Could you check a few things on this model? Use its own coordinates, in mm. A direction names the side the tool comes from. Give positions to 0.01 mm unless a question says otherwise; leave off trailing zeros. Loops run counter-clockwise (first coordinate to the right, second up) from the corner with the lowest first, then second, coordinate; pieces in that order, holes last. Notation, with made-up numbers: M 82.25,-7 L 137.25,-7 A34 cw 137.25,27 Z; hole C 76.5,84 d4. An arc over 180 degrees is marked long. Return JSON: item names as keys, results as strings. Group by question number.
1. Please list where these lines run through material, in increasing order: line 1 (X direction, y = -60, z = 45); line 2 (Z direction, x = 15, y = -59); line 3 (Z direction, x = 19.5, y = -23).
2. If we mould it in two halves opening along X, with no side actions, what happens to faces 3 (the cylindrical face through (1, -37, 2)), 4 (the flat face through (15, -20, 68)), 5 (the cylindrical face through (94.06, -37.53, 1.43)), 6 (the flat face through (47, -49, 0))? For each: +X half, -X half, draft (parallel to the pull), parting line (faces both ways), or undercut.
3. For pin 1 (22 mm diameter, centred on x = 68.5, z = 61.5, fed in from -Y); pin 2 (7.5 mm diameter, centred on x = 41, z = 45.5, fed in from -Y); pin 3 (17 mm diameter, centred on x = 15, z = 45, fed in from -Y), each with a flat end and sliding along its axis, tell me the tip position at first contact or that it passes through.
4. If we section it at D-D (x = 15): Write out the boundary of the cut face in (y, z), plus the area to 3 significant figures.
5. If we section it at B-B (z = 57): Write out the boundary of the cut face in (x, y), plus the area to 3 significant figures.
6. If we section it at C-C (x = 41): Write out the boundary of the cut face in (y, z), plus the area to 3 significant figures.
7. If we section it at A-A (y = -62.5): Write out the boundary of the cut face in (x, z), plus the area to 3 significant figures.
8. For faces 1 (the flat face through (27.28, -87.13, 44.37)), 2 (the flat face through (15, -20, 45)), which set-ups out of +Z, -Z, +X, -X, +Y, -Y let a thin tool reach every point of the face, with its end or its side?
```python
from build123d import *

# Parameters (mm, degrees)
F0_W        = 95.5598546359
F0_H        = 90
F1_DEPTH    = 100
F2_R        = 5
F3_W        = 20
F3_H        = 70
F3_R        = 7.5
F4_DEPTH    = 80
F5_T1_DEPTH = 92.4997500025
F7_DEPTH    = 90
F8_T1_DEPTH = 105.435292613


# Not quite as in the source:
# - a fillet or chamfer that OpenCascade refuses, or shapes differently, is made with other operations: its cross-section is extruded or revolved along the edge and cut away or added


with BuildPart() as f1:
    # F0 (on Front) → F1 (new body)
    with BuildSketch(Plane.XZ):
        with Locations((47.7799273179, 45)):
            Rectangle(F0_W, F0_H)
    extrude(amount=F1_DEPTH)

    # F2
    f2_edges = [f1.edges().sort_by_distance(p)[0] for p in [
        (95.559855, -50, 90),
        (95.559855, -50, 0),
        (0, -50, 0),
        (0, -50, 90),
    ]]
    fillet(f2_edges, radius=F2_R)

    # F3 (on face) → F4 (cut)
    with BuildSketch(Plane.XZ.offset(100)):
        with Locations((73.0598546359, 45)):
            Rectangle(F3_W, F3_H)
        with Locations((15, 45)):
            Circle(F3_R)
        with Locations((15, 68)):
            Circle(F3_R)
        with Locations((40, 45)):
            Circle(F3_R)
        with Locations((40, 68)):
            Circle(F3_R)
        with Locations((15, 20)):
            Circle(F3_R)
        with Locations((40, 20)):
            Circle(F3_R)
    extrude(amount=-F4_DEPTH, mode=Mode.SUBTRACT)

    # F5: fillet of radius 5 on 4 edges, made by hand

    # F5_s2 → F5_t1 (join)
    with BuildSketch(Plane.XZ.offset(7.5002499975)):
        with BuildLine():
            ThreePointArc((68.0597546359, 80.0001), (64.5242207299, 78.5356339059), (63.0597546359, 75.0001))
            Line((63.0597546359, 75.0001), (62.9597546359, 75.0001))
            ThreePointArc((62.9597546359, 75.0001), (62.9598546359, 77.50005), (62.9598546359, 80))
            Line((62.9598546359, 80), (63.0598546359, 80.1))
            ThreePointArc((63.0598546359, 80.1), (65.5598046359, 80.1), (68.0597546359, 80.1001))
            Line((68.0597546359, 80.1001), (68.0597546359, 80.0001))
        make_face()
        with BuildLine():
            ThreePointArc((78.0599546359, 80.0001), (81.5954885418, 78.5356339059), (83.0599546359, 75.0001))
            Line((83.0599546359, 75.0001), (83.1599546359, 75.0001))
            ThreePointArc((83.1599546359, 75.0001), (83.1598546359, 77.50005), (83.1598546359, 80))
            Line((83.1598546359, 80), (83.0598546359, 80.1))
            ThreePointArc((83.0598546359, 80.1), (80.5599046359, 80.1), (78.0599546359, 80.1001))
            Line((78.0599546359, 80.1001), (78.0599546359, 80.0001))
        make_face()
        with BuildLine():
            ThreePointArc((78.0599546359, 9.9999), (81.5954885418, 11.4643660941), (83.0599546359, 14.9999))
            Line((83.0599546359, 14.9999), (83.1599546359, 14.9999))
            ThreePointArc((83.1599546359, 14.9999), (83.1598546359, 12.49995), (83.1598546359, 10))
            Line((83.1598546359, 10), (83.0598546359, 9.9))
            ThreePointArc((83.0598546359, 9.9), (80.5599046359, 9.9), (78.0599546359, 9.8999))
            Line((78.0599546359, 9.8999), (78.0599546359, 9.9999))
        make_face()
        with BuildLine():
            ThreePointArc((63.0597546359, 14.9999), (64.5242207299, 11.4643660941), (68.0597546359, 9.9999))
            Line((68.0597546359, 9.9999), (68.0597546359, 9.8999))
            ThreePointArc((68.0597546359, 9.8999), (65.5598046359, 9.9), (63.0598546359, 9.9))
            Line((63.0598546359, 9.9), (62.9598546359, 10))
            ThreePointArc((62.9598546359, 10), (62.9598546359, 12.49995), (62.9597546359, 14.9999))
            Line((62.9597546359, 14.9999), (63.0597546359, 14.9999))
        make_face()
    extrude(amount=F5_T1_DEPTH)

    # F6 (on face) → F7 (cut)
    with BuildSketch(Plane(origin=(0, 0, 0), x_dir=(1, 0, 0), z_dir=(0, 0, -1))):
        Polygon((0, 124.7042194009), (0, 70), (47.7799273179, 100), (97.1999242902, 70), (97.1999242902, 124.7042194009), align=None)
    extrude(amount=-F7_DEPTH, mode=Mode.SUBTRACT)

    # F8: fillet of radius 5 on 1 edges, made by hand

    # F8_s2 → F8_t1 (cut)
    with BuildSketch(Plane.XY.offset(-7.7176463065)):
        with BuildLine():
            ThreePointArc((45.1654951007, -98.3584536244), (47.7865363785, -99.1238075774), (50.4188247907, -98.3980791373))
            Line((50.4188247907, -98.3980791373), (47.7799273179, -100))
            Line((47.7799273179, -100), (45.1654951007, -98.3584536244))
        make_face()
    extrude(amount=F8_T1_DEPTH, mode=Mode.SUBTRACT)


solid = f1.part
```
Answer:
{
 "1": {"line 1": "x = 0 to 7.5, 22.5 to 32.5, 47.5 to 63.06, 83.06 to 95.56", "line 2": "z = 0 to 12.5, 27.5 to 37.5, 52.5 to 60.5, 75.5 to 90", "line 3": "z = 0 to 14, 26 to 39, 51 to 62, 74 to 90"},
 "2": {"face 3": "-X half", "face 4": "undercut", "face 5": "+X half", "face 6": "draft"},
 "3": {"pin 1": "stops at y = -94.1", "pin 2": "stops at y = -20", "pin 3": "stops at y = -84.76"},
 "4": {"outline": "M -79.42,0 L 0,0 L 0,90 L -79.42,90 L -79.42,75.5 L -20,75.5 L -20,60.5 L -79.42,60.5 L -79.42,52.5 L -20,52.5 L -20,37.5 L -79.42,37.5 L -79.42,27.5 L -20,27.5 L -20,12.5 L -79.42,12.5 Z", "area": "4,470 mm²"},
 "5": {"outline": "M 0,-70 L 45.17,-98.36 A5 ccw 50.42,-98.4 L 63.06,-90.72 L 63.06,-20 L 83.06,-20 L 83.06,-78.58 L 95.56,-71 L 95.56,0 L 0,0 Z", "area": "6,850 mm²"},
 "6": {"outline": "M -95.74,0 L 0,0 L 0,90 L -95.74,90 L -95.74,75.43 L -20,75.43 L -20,60.57 L -95.74,60.57 L -95.74,52.43 L -20,52.43 L -20,37.57 L -95.74,37.57 L -95.74,27.43 L -20,27.43 L -20,12.57 L -95.74,12.57 Z", "area": "5,240 mm²"},
 "7": {"outline": "M 0,5 A5 ccw 5,0 L 90.56,0 A5 ccw 95.56,5 L 95.56,85 A5 ccw 90.56,90 L 5,90 A5 ccw 0,85 Z; hole C 15,20 d15; hole C 15,45 d15; hole C 15,68 d15; hole C 40,20 d15; hole C 40,45 d15; hole C 40,68 d15; hole M 63.06,14.97 A5 ccw 68.03,10 L 78.09,10 A5 ccw 83.06,14.97 L 83.06,75.03 A5 ccw 78.09,80 L 68.03,80 A5 ccw 63.06,75.03 Z", "area": "6,140 mm²"},
 "8": {"face 1": "+Z, -Z, -X, -Y", "face 2": "-Y"}
}
